from build123d import *

# Parameters (mm, degrees)
F0_W     = 7.62
F0_H     = 15.875
F1_DEPTH = 4.7625
F2_R     = 2.4511
F3_DEPTH = 1.778
F4_W     = 4.572
F4_H     = 12.827
F5_DEPTH = 8.382
F7_DEPTH = 7.77


with BuildPart() as f1:
    # F0 (on Top) → F1 (new body, symmetric)
    with BuildSketch(Plane.XY):
        Rectangle(F0_W, F0_H)
    extrude(amount=F1_DEPTH, both=True)

    # F2 (on face) → F3 (join)
    with BuildSketch(Plane.XY.offset(4.7625)):
        with Locations((0, 4.0132)):
            Circle(F2_R)
        with Locations((0, -4.0132)):
            Circle(F2_R)
    extrude(amount=F3_DEPTH)

    # F4 (on face) → F5 (cut)
    with BuildSketch(Plane(origin=(0, 0, -4.7625), x_dir=(1, 0, 0), z_dir=(0, 0, -1))):
        Rectangle(F4_W, F4_H)
    extrude(amount=-F5_DEPTH, mode=Mode.SUBTRACT)

    # F6 (on face) → F7 (cut)
    with BuildSketch(Plane.YZ.offset(3.81)):
        Polygon((1.302941, 3.120179), (-0.697059, 3.120179), (-0.697059, 1.120179), (-2.697059, 1.120179), (-2.697059, -0.879821), (-0.697059, -0.879821), (-0.697059, -2.879821), (1.302941, -2.879821), (1.302941, -0.879821), (3.302941, -0.879821), (3.302941, 1.120179), (1.302941, 1.120179), align=None)
    extrude(amount=-F7_DEPTH, mode=Mode.SUBTRACT)


solid = f1.part
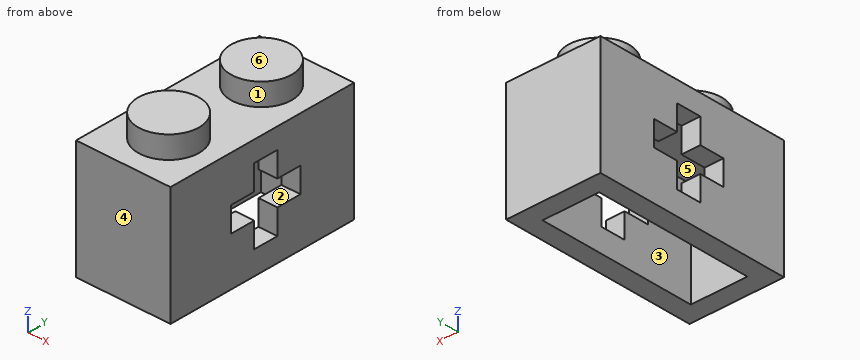
Geometry check sheet. Reference: the model listing, model coordinates, mm. Face numbers are marked on the shaded views. A direction names the side the tool comes from. Give positions to 0.01 mm unless a question says otherwise; leave off trailing zeros. Order: outer loops, then holes, each group sorted by start corner. A loop starts at its lowest first (then second) coordinate and runs counter-clockwise, first axis right, second up. Notation, with made-up numbers: (47.25, 82.25) - (88.25, 82.25) arc R20 ccw to (88.25, 116.25) - close; hole circle Ø6 at (-0.5, 87.5). An arc over 180 degrees is marked (long way). Answer as a JSON object with one key per item and string values.
(1) Tool access check on the marked faces 1, 2 and 3. Record the directions out of +Z, -Z, +X, -X, +Y, -Y that give a thin tool (end or side, any length) a straight path to the whole face; none if there is none.
Report:
{"face 1": "+Z", "face 2": "+X, -X", "face 3": "-Z"}
(2) Material ranges on line 1 (X direction, y = -6, z = 2.5); line 2 (Y direction, x = 1.25, z = -0.25); line 3 (Y direction, x = -3, z = -0.5), recorded low to high.
Report:
{"line 1": "-3.81 to -2.29, 2.29 to 3.81", "line 2": "-7.94 to -6.41, 6.41 to 7.94", "line 3": "-7.94 to -2.7, 3.3 to 7.94"}
(3) Draft check along Y on the marked faces 4, 5 and 6. Enter one of: released by +Y, released by -Y, zero draft, split by the parting line, or undercut.
Report:
{"face 4": "released by -Y", "face 5": "undercut", "face 6": "zero draft"}
(4) Depth check by flat-ended pin: pin 1 Ø1.2 at (x, y) = (-3.5, -2) entering from +Z. Enter the tip coordinate at first touch or a pass-through.
Report:
{"pin 1": "z = 4.76"}
(5) Cross-section at B-B (y = 0). Record the cut outline in (x, z), then the cut area to 3 significant figures.
Report:
{"outline": "(-3.81, -4.76) - (-2.29, -4.76) - (-2.29, -2.88) - (-3.81, -2.88) - close; (-3.81, 3.12) - (-2.29, 3.12) - (-2.29, 3.62) - (2.29, 3.62) - (2.29, 3.12) - (3.81, 3.12) - (3.81, 4.76) - (-3.81, 4.76) - close; (2.29, -4.76) - (3.81, -4.76) - (3.81, -2.88) - (2.29, -2.88) - close", "area": "16.0 mm^2"}
(6) Cross-section at A-A (z = 1.5). Record the cut outline in (x, y).
Report:
{"outline": "(-3.81, -7.94) - (3.81, -7.94) - (3.81, -0.7) - (2.29, -0.7) - (2.29, -6.41) - (-2.29, -6.41) - (-2.29, -0.7) - (-3.81, -0.7) - close; (-3.81, 1.3) - (-2.29, 1.3) - (-2.29, 6.41) - (2.29, 6.41) - (2.29, 1.3) - (3.81, 1.3) - (3.81, 7.94) - (-3.81, 7.94) - close"}
(7) Cross-section at D-D (z = -3.25). Record the cut outline in (x, y), then the cut area to 3 significant figures.
Report:
{"outline": "(-3.81, -7.94) - (3.81, -7.94) - (3.81, 7.94) - (-3.81, 7.94) - close; hole (-2.29, -6.41) - (2.29, -6.41) - (2.29, 6.41) - (-2.29, 6.41) - close", "area": "62.3 mm^2"}
(8) Cross-section at C-C (x = 0). Record the cut outline in (y, z).
Report:
{"outline": "(-7.94, -4.76) - (-6.41, -4.76) - (-6.41, 3.62) - (6.41, 3.62) - (6.41, -4.76) - (7.94, -4.76) - (7.94, 4.76) - (6.46, 4.76) - (6.46, 6.54) - (1.56, 6.54) - (1.56, 4.76) - (-1.56, 4.76) - (-1.56, 6.54) - (-6.46, 6.54) - (-6.46, 4.76) - (-7.94, 4.76) - close"}
